from build123d import *

# Parameters (mm, degrees)
SKETCH1_R           = 227.5
BOSS_EXTRUDE1_DEPTH = 7.5
BOSS_EXTRUDE2_START = 7.5
SKETCH1_3_R         = 15
BOSS_EXTRUDE2_DEPTH = 35
SKETCH2_R           = 40
SKETCH2_R_2         = 30
CUT_EXTRUDE1_DEPTH  = 16
CUT_EXTRUDE3_START  = 7.5
SKETCH3_R           = 15
CUT_EXTRUDE3_DEPTH  = 15


with BuildPart() as part:
    # Sketch1 → Boss-Extrude1 (new body, symmetric)
    with BuildSketch(Plane.XY):
        Circle(SKETCH1_R)
    extrude(amount=BOSS_EXTRUDE1_DEPTH, both=True)

    # Sketch1<3> → Boss-Extrude2 (add)
    with BuildSketch(Plane.XY.offset(BOSS_EXTRUDE2_START)):
        with Locations((0, 200)):
            Circle(SKETCH1_3_R)
    extrude(amount=BOSS_EXTRUDE2_DEPTH)

    # Sketch2 → Cut-Extrude1 (cut, through all)
    with BuildSketch(Plane.XY.offset(7.5)):
        with Locations((-172.341356777, 30.388431092)):
            Circle(SKETCH2_R)
        with Locations((0, 100)):
            Circle(SKETCH2_R_2)
        with Locations((90.630778704, 42.261826174)):
            Circle(SKETCH2_R_2)
        with Locations((-90.630778704, -42.261826174)):
            Circle(SKETCH2_R_2)
        with Locations((112.487831695, 134.057777546)):
            Circle(SKETCH2_R)
        with Locations((59.853525082, -164.446208638)):
            Circle(SKETCH2_R)
    extrude(amount=-CUT_EXTRUDE1_DEPTH, mode=Mode.SUBTRACT)

    # Sketch3 → Cut-Extrude3 (cut)
    with BuildSketch(Plane.XY.offset(CUT_EXTRUDE3_START)):
        Circle(SKETCH3_R)
    extrude(amount=-CUT_EXTRUDE3_DEPTH, mode=Mode.SUBTRACT)


solid = part.part
For this review, take the finished solid that the model builds, in its own axes (mm). A direction names the side the tool comes from. Give positions to 0.01 mm unless a question says otherwise; leave off trailing zeros. Loops run counter-clockwise (first coordinate to the right, second up) from the corner with the lowest first, then second, coordinate; pieces in that order, holes last.
Item 1: Insertion check: pin 1 (12 mm diameter, centred on x = -139, y = 41.5, fed in from -Z); pin 2 (1.5 mm diameter, centred on y = 108.5, z = 4, fed in from -X); pin 3 (10 mm diameter, centred on x = 21.5, z = -2, fed in from +Y); pin 4 (1 mm diameter, centred on x = 14, y = 13, fed in from +Z). Each pin has a flat end and moves straight along its axis. Give the tip position at first contact, or say it passes through.
Item 2: For line 1 along Z through (x, y) = (-158.5, -99.5); line 2 along X through (y, z) = (111, 3.5); line 3 along X through (y, z) = (87.5, 4.5), list the stretches that pass through material, from the lowest coordinate up.
Item 3: Draft analysis for pull direction X (two halves, no side actions). For faces 1 (the cylindrical face through (119.245, 51.273, 0.105)), 2 (the cylindrical face through (-3.905, 129.745, 0.105)), 3 (the flat face through (-3, -47, 7.5)), 4 (the cylindrical face through (216.994, 68.335, 0.105)), state which applies: +X half, -X half, draft (parallel to the pull), parting line (faces both ways), or undercut.
Item 4: Take a section at C-C, the plane z = 1. State the section outline as (x, y) points, and give its area (3 significant figures).
Item 5: Take a section at D-D, the plane y = 0. State the section outline as (x, z) points.
Item 6: Take a section at A-A, the plane x = 0. State the section outline as (y, z) points.
Item 7: Tool access review of faces 5 (the cylindrical face through (-3.252, 185.357, 24.755)), 6 (the cylindrical face through (-212.303, 32.147, 0.105)): name each direction out of +Z, -Z, +X, -X, +Y, -Y from which nothing blocks a thin tool from reaching the whole face with its end or side.
Item 8: Take a section at B-B, the plane y = 86. State the section outline as (x, z) points.
Calculated:
1. pin 1: stops at z = -7.5
1. pin 2: stops at x = -200.37
1. pin 3: stops at y = 226.9
1. pin 4: stops at z = 7.5
2. line 1: z = -7.5 to 7.5
2. line 2: x = -198.58 to -27.91, 27.91 to 79.8, 145.17 to 198.58
2. line 3: x = -210 to -27.27, 27.27 to 210
3. face 1: undercut
3. face 2: undercut
3. face 3: draft
3. face 4: parting line
4. outline: circle Ø455 at (0, 0); hole circle Ø80 at (-172.34, 30.39); hole circle Ø60 at (-90.63, -42.26); hole circle Ø60 at (0, 100); hole circle Ø30 at (0, 0); hole circle Ø80 at (59.85, -164.45); hole circle Ø60 at (90.63, 42.26); hole circle Ø80 at (112.49, 134.06)
4. area: 138,000 mm2
5. outline: (-227.5, -7.5) - (-198.35, -7.5) - (-198.35, 7.5) - (-227.5, 7.5) - close; (-146.33, -7.5) - (-15, -7.5) - (-15, 7.5) - (-146.33, 7.5) - close; (15, -7.5) - (227.5, -7.5) - (227.5, 7.5) - (15, 7.5) - close
6. outline: (-227.5, -7.5) - (-15, -7.5) - (-15, 7.5) - (-227.5, 7.5) - close; (15, -7.5) - (70, -7.5) - (70, 7.5) - (15, 7.5) - close; (130, -7.5) - (227.5, -7.5) - (227.5, 7.5) - (215, 7.5) - (215, 42.5) - (185, 42.5) - (185, 7.5) - (130, 7.5) - close
7. face 5: +Z
7. face 6: +Z, -Z
8. outline: (-210.62, -7.5) - (-26.53, -7.5) - (-26.53, 7.5) - (-210.62, 7.5) - close; (26.53, -7.5) - (210.62, -7.5) - (210.62, 7.5) - (26.53, 7.5) - close
